Design review of the part built by this model. Coordinates are the model's own, in mm. Coordinates: 2 decimals unless noted, no trailing zeros. Order: outer loops, then holes, each group sorted by start corner. A loop starts at its lowest first (then second) coordinate and runs counter-clockwise, first axis right, second up. Notation, with made-up numbers: (26.25, -21) - (68.25, -21) arc R24 cw to (68.25, -11) - close; hole circle Ø9 at (-28, 16). An arc over 180 degrees is marked (long way). Write item = value, one per line. Start each with the question number.
```python
from build123d import *

# Parameters (mm, degrees)
SKETCH1_R           = 30
SKETCH1_R_2         = 1.4224
BOSS_EXTRUDE1_DEPTH = 2.54


with BuildPart() as part:
    # Sketch1 → Boss-Extrude1 (new body)
    with BuildSketch(Plane(origin=(0, 0, 0), x_dir=(1, 0, 0), z_dir=(0, 1, 0))):
        Circle(SKETCH1_R)
        with Locations((6.35, 0)):
            Circle(SKETCH1_R_2, mode=Mode.SUBTRACT)
        with Locations((-6.35, 0)):
            Circle(SKETCH1_R_2, mode=Mode.SUBTRACT)
        with BuildLine():
            Line((-1.905, 24.927313873), (-1.905, 12.027696635))
            Line((-1.905, 12.027696635), (-5.891200947, 24.295961666))
            ThreePointArc((-5.891200947, 24.295961666), (-3.910861632, 24.692208552), (-1.905, 24.927313873))
        make_face(mode=Mode.SUBTRACT)
        with BuildLine():
            Line((1.905, 24.927313873), (1.905, 12.027696635))
            Line((1.905, 12.027696635), (5.891200947, 24.295961666))
            ThreePointArc((5.891200947, 24.295961666), (3.910861632, 24.692208552), (1.905, 24.927313873))
        make_face(mode=Mode.SUBTRACT)
        with BuildLine():
            Line((9.514726274, 23.118606918), (5.528525327, 10.850341887))
            Line((5.528525327, 10.850341887), (13.110730099, 21.286351453))
            ThreePointArc((13.110730099, 21.286351453), (11.349762511, 22.275163139), (9.514726274, 23.118606918))
        make_face(mode=Mode.SUBTRACT)
        with BuildLine():
            Line((16.193084848, 19.046889641), (8.610880076, 8.610880076))
            Line((8.610880076, 8.610880076), (19.046889641, 16.193084848))
            ThreePointArc((19.046889641, 16.193084848), (17.677669557, 17.677669557), (16.193084848, 19.046889641))
        make_face(mode=Mode.SUBTRACT)
        with BuildLine():
            Line((21.286351453, 13.110730099), (10.850341887, 5.528525327))
            Line((10.850341887, 5.528525327), (23.118606918, 9.514726274))
            ThreePointArc((23.118606918, 9.514726274), (22.275163139, 11.349762511), (21.286351453, 13.110730099))
        make_face(mode=Mode.SUBTRACT)
        with BuildLine():
            Line((24.295961666, 5.891200947), (12.027696635, 1.905))
            Line((12.027696635, 1.905), (24.927313873, 1.905))
            ThreePointArc((24.927313873, 1.905), (24.692208552, 3.910861632), (24.295961666, 5.891200947))
        make_face(mode=Mode.SUBTRACT)
        with BuildLine():
            Line((24.927313873, -1.905), (12.027696635, -1.905))
            Line((12.027696635, -1.905), (24.295961666, -5.891200947))
            ThreePointArc((24.295961666, -5.891200947), (24.692208552, -3.910861632), (24.927313873, -1.905))
        make_face(mode=Mode.SUBTRACT)
        with BuildLine():
            Line((23.118606918, -9.514726274), (10.850341887, -5.528525327))
            Line((10.850341887, -5.528525327), (21.286351453, -13.110730099))
            ThreePointArc((21.286351453, -13.110730099), (22.275163139, -11.349762511), (23.118606918, -9.514726274))
        make_face(mode=Mode.SUBTRACT)
        with BuildLine():
            Line((19.046889641, -16.193084848), (8.610880076, -8.610880076))
            Line((8.610880076, -8.610880076), (16.193084848, -19.046889641))
            ThreePointArc((16.193084848, -19.046889641), (17.677669557, -17.677669557), (19.046889641, -16.193084848))
        make_face(mode=Mode.SUBTRACT)
        with BuildLine():
            Line((13.110730099, -21.286351453), (5.528525327, -10.850341887))
            Line((5.528525327, -10.850341887), (9.514726274, -23.118606918))
            ThreePointArc((9.514726274, -23.118606918), (11.349762511, -22.275163139), (13.110730099, -21.286351453))
        make_face(mode=Mode.SUBTRACT)
        with BuildLine():
            Line((5.891200947, -24.295961666), (1.905, -12.027696635))
            Line((1.905, -12.027696635), (1.905, -24.927313873))
            ThreePointArc((1.905, -24.927313873), (3.910861632, -24.692208552), (5.891200947, -24.295961666))
        make_face(mode=Mode.SUBTRACT)
        with BuildLine():
            Line((-1.905, -24.927313873), (-1.905, -12.027696635))
            Line((-1.905, -12.027696635), (-5.891200947, -24.295961666))
            ThreePointArc((-5.891200947, -24.295961666), (-3.910861632, -24.692208552), (-1.905, -24.927313873))
        make_face(mode=Mode.SUBTRACT)
        with BuildLine():
            Line((-9.514726274, -23.118606918), (-5.528525327, -10.850341887))
            Line((-5.528525327, -10.850341887), (-13.110730099, -21.286351453))
            ThreePointArc((-13.110730099, -21.286351453), (-11.349762511, -22.275163139), (-9.514726274, -23.118606918))
        make_face(mode=Mode.SUBTRACT)
        with BuildLine():
            Line((-16.193084848, -19.046889641), (-8.610880076, -8.610880076))
            Line((-8.610880076, -8.610880076), (-19.046889641, -16.193084848))
            ThreePointArc((-19.046889641, -16.193084848), (-17.677669557, -17.677669557), (-16.193084848, -19.046889641))
        make_face(mode=Mode.SUBTRACT)
        with BuildLine():
            Line((-21.286351453, -13.110730099), (-10.850341887, -5.528525327))
            Line((-10.850341887, -5.528525327), (-23.118606918, -9.514726274))
            ThreePointArc((-23.118606918, -9.514726274), (-22.275163139, -11.349762511), (-21.286351453, -13.110730099))
        make_face(mode=Mode.SUBTRACT)
        with BuildLine():
            Line((-24.295961666, -5.891200947), (-12.027696635, -1.905))
            Line((-12.027696635, -1.905), (-24.927313873, -1.905))
            ThreePointArc((-24.927313873, -1.905), (-24.692208552, -3.910861632), (-24.295961666, -5.891200947))
        make_face(mode=Mode.SUBTRACT)
        with BuildLine():
            Line((-24.927313873, 1.905), (-12.027696635, 1.905))
            Line((-12.027696635, 1.905), (-24.295961666, 5.891200947))
            ThreePointArc((-24.295961666, 5.891200947), (-24.692208552, 3.910861632), (-24.927313873, 1.905))
        make_face(mode=Mode.SUBTRACT)
        with BuildLine():
            Line((-23.118606918, 9.514726274), (-10.850341887, 5.528525327))
            Line((-10.850341887, 5.528525327), (-21.286351453, 13.110730099))
            ThreePointArc((-21.286351453, 13.110730099), (-22.275163139, 11.349762511), (-23.118606918, 9.514726274))
        make_face(mode=Mode.SUBTRACT)
        with BuildLine():
            Line((-19.046889641, 16.193084848), (-8.610880076, 8.610880076))
            Line((-8.610880076, 8.610880076), (-16.193084848, 19.046889641))
            ThreePointArc((-16.193084848, 19.046889641), (-17.677669557, 17.677669557), (-19.046889641, 16.193084848))
        make_face(mode=Mode.SUBTRACT)
        with BuildLine():
            Line((-13.110730099, 21.286351453), (-5.528525327, 10.850341887))
            Line((-5.528525327, 10.850341887), (-9.514726274, 23.118606918))
            ThreePointArc((-9.514726274, 23.118606918), (-11.349762511, 22.275163139), (-13.110730099, 21.286351453))
        make_face(mode=Mode.SUBTRACT)
    extrude(amount=BOSS_EXTRUDE1_DEPTH)


solid = part.part
```
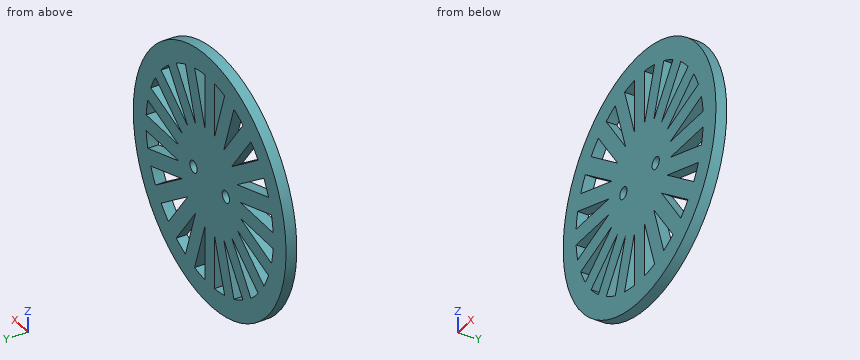
Item 1: For P1, Ø1.3, axis at y = 1.5, z = 15.5, coming from the +X side; P2, Ø0.8, axis at x = 20, y = 1.5, coming from the -Z side; P3, Ø1.5, axis at y = 1, z = -15, coming from the +X side, all flat-tipped, find the tip position at first contact; note any pin that passes through.
Item 2: For line 1 (X direction, y = 1.4, z = 0); line 2 (X direction, y = 1.35, z = -22) (3 decimals); line 3 (Z direction, x = -10, y = 0.25), list the stretches that pass through material, from the lowest coordinate up.
Item 3: Add section B-B on y = 1.45. State how many separate pieces and enclosed holes the cut face has, plus the area to 3 significant figures.
Item 4: Add section A-A on z = 0. Give the boundary of the cut face in (x, y).
Worked out:
q1.P1 = 26.07
q1.P2 = -22.71
q1.P3 = 26.4
q2.line_1 = -30 to -7.77, -4.93 to 4.93, 7.77 to 30
q2.line_2 = -20.396 to -11.874, -9.151 to -5.145, -1.905 to 1.905, 5.145 to 9.151, 11.874 to 20.396
q2.line_3 = -28.28 to -22.91, -17 to -10.52, -9.62 to 9.62, 10.52 to 17, 22.91 to 28.28
q3.separate_pieces = 1
q3.enclosed_holes = 22
q3.area = 2,300 mm2
q4.outline = (-30, 0) - (-7.77, 0) - (-7.77, 2.54) - (-30, 2.54) - close; (-4.93, 0) - (4.93, 0) - (4.93, 2.54) - (-4.93, 2.54) - close; (7.77, 0) - (30, 0) - (30, 2.54) - (7.77, 2.54) - close
